Here's how the part is built. I have some questions about the finished solid (model axes, mm). Face numbers are marked on the shaded views. A direction names the side the tool comes from. Coordinates: 2 decimals unless noted, no trailing zeros. Order: outer loops, then holes, each group sorted by start corner. A loop starts at its lowest first (then second) coordinate and runs counter-clockwise, first axis right, second up. Notation, with made-up numbers: (23.25, 27.5) - (38.25, 27.5) arc R28 cw to (38.25, 48.5) - close; hole circle Ø10 at (85, -3). An arc over 180 degrees is marked (long way). Answer in a Markdown table with one row per item. Add a question column.
Item 1: Thinking about a two-plate mould opening in Y: for the marked faces 1, 2 and 3, which applies, +Y half, -Y half, draft (parallel to the pull), parting line (faces both ways), or undercut?
Item 2: On a 3-axis mill with a long thin cutter (end or side, diameter ignored), from which of +Z, -Z, +X, -X, +Y, -Y can I reach the whole of each face in a straight line? I mean the marked faces 4 and 5. Say none if no direction works.
Item 3: I want a section at D-D (y = 19.05). Please give me the cut outline in (x, z) (3 decimals), plus the area to 3 significant figures.
Item 4: If I drill on line 1 along Y through (x, z) = (26.5, -3) (3 decimals); line 2 along Z through (x, y) = (1, -0.5) (3 decimals); line 3 along X through (y, z) = (3.5, 2.5), over which ranges is the centre line in solid material (lowest first)? Write a range as from..to.
Item 5: I want a section at A-A (x = -7). Please give me the cut outline in (y, z) (3 decimals).
Item 6: I want a section at B-B (x = -25.4). Please give me the cut outline in (y, z) (1 decimal).
Item 7: I want a section at C-C (y = 4). Please give me the cut outline in (x, z) (3 decimals), plus the area to 3 significant figures.
Item 8: Will these pins go through, and if not, where does the flat tip stop? pin 1 Ø2 at (x, z) = (19.05, -2.38) entering from +Y; pin 2 Ø1.6 at (y, z) = (-29.5, -1.5) entering from -X (3 decimals); pin 3 Ø4.5 at (x, y) = (-25.4, 19.05) entering from -Z (3 decimals); pin 4 Ø3 at (x, z) = (19.05, -2.38) entering from -Y.
```python
from build123d import *

# Parameters (mm, degrees)
SKETCH1_W                 = 63.5
SKETCH1_H                 = 63.5
BOSS_EXTRUDE1_DEPTH       = 3.175
BOSS_EXTRUDE2_DEPTH       = 4.7625
F_2_CLEARANCE_HOLE1_D     = 2.4384
F_2_CLEARANCE_HOLE1_DEPTH = 3.175
FILLET1_R                 = 19.05
SKETCH5_W                 = 15.875
SKETCH5_H                 = 3.175
BOSS_EXTRUDE3_DEPTH       = 4.7625
F_2_CLEARANCE_HOLE2_D     = 2.4384
F_2_CLEARANCE_HOLE2_DEPTH = 3.175
BOSS_EXTRUDE4_START       = -3.175
SKETCH8_R                 = 3.175
BOSS_EXTRUDE4_DEPTH       = 3.175
F_6_CLEARANCE_HOLE1_D     = 3.7973
CUT_EXTRUDE1_REACH        = 9.938
SKETCH11_R                = 3.175


with BuildPart() as part:
    # Sketch1 → Boss-Extrude1 (new body)
    with BuildSketch(Plane.XY):
        Rectangle(SKETCH1_W, SKETCH1_H)
    extrude(amount=BOSS_EXTRUDE1_DEPTH)

    # Sketch2 → Boss-Extrude2 (add)
    with BuildSketch(Plane(origin=(0, 0, 0), x_dir=(-1, 0, 0), z_dir=(0, 0, -1))):
        Polygon((-25.4, -31.75), (-15.875, -31.75), (-15.875, -28.575), (-25.4, -28.575), (-31.75, -28.575), (-31.75, -31.75), align=None)
    extrude(amount=BOSS_EXTRUDE2_DEPTH)

    # #2 Clearance Hole1
    with Locations(Plane(origin=(0, -28.575, 0), x_dir=(1, 0, 0), z_dir=(0, 1, 0))):
        with Locations((28.575, 2.38125), (19.05, 2.38125)):
            Hole(F_2_CLEARANCE_HOLE1_D / 2, depth=F_2_CLEARANCE_HOLE1_DEPTH)

    # Fillet1
    fillet1_edges = [part.edges().sort_by_distance(p)[0] for p in [
        (-31.75, -31.75, 1.5875),
        (-31.75, 31.75, 1.5875),
    ]]
    fillet(fillet1_edges, radius=FILLET1_R)

    # Sketch5 → Boss-Extrude3 (add)
    with BuildSketch(Plane(origin=(0, 0, 0), x_dir=(-1, 0, 0), z_dir=(0, 0, -1))):
        with Locations((-23.8125, 30.1625)):
            Rectangle(SKETCH5_W, SKETCH5_H)
    extrude(amount=BOSS_EXTRUDE3_DEPTH)

    # #2 Clearance Hole2
    with Locations(Plane(origin=(0, 28.575, 0), x_dir=(-1, 0, 0), z_dir=(0, -1, 0))):
        with Locations((-19.05, 2.38125), (-28.575, 2.38125)):
            Hole(F_2_CLEARANCE_HOLE2_D / 2, depth=F_2_CLEARANCE_HOLE2_DEPTH)

    # Sketch8 → Boss-Extrude4 (add)
    with BuildSketch(Plane.XY.offset(3.175).offset(BOSS_EXTRUDE4_START)):
        with Locations((-25.4, 19.05)):
            Circle(SKETCH8_R)
        with Locations((-25.4, -14.2875)):
            Circle(SKETCH8_R)
        with Locations((22.225, 19.05)):
            Circle(SKETCH8_R)
        with Locations((8.73125, -24.209375)):
            Circle(SKETCH8_R)
        with Locations((-11.90625, -24.209375)):
            Circle(SKETCH8_R)
    extrude(amount=-BOSS_EXTRUDE4_DEPTH)

    # #6 Clearance Hole1 (through all)
    with Locations(Plane(origin=(0, 0, -3.175), x_dir=(-1, 0, 0), z_dir=(0, 0, -1))):
        with Locations((-22.225, 19.05), (25.4, 19.05), (25.4, -14.2875), (11.90625, -24.209375), (-8.73125, -24.209375)):
            Hole(F_6_CLEARANCE_HOLE1_D / 2)

    # Sketch11 → Cut-Extrude1 (cut, up to next)
    with BuildSketch(Plane.XY.offset(3.175), mode=Mode.PRIVATE) as cut_extrude1_sk1:
        with Locations((-1.5875, -23.415625)):
            Circle(SKETCH11_R)
    cut_extrude1_tool1 = extrude(cut_extrude1_sk1.sketch, amount=-CUT_EXTRUDE1_REACH, mode=Mode.PRIVATE) & part.part
    add(cut_extrude1_tool1.solids().sort_by_distance((-1.5875, -23.415625, 3.175))[0], mode=Mode.SUBTRACT)
    # Sketch11 → Cut-Extrude1 (cut, up to next)
    with BuildSketch(Plane.XY.offset(3.175), mode=Mode.PRIVATE) as cut_extrude1_sk2:
        with BuildLine():
            Line((-4.7625, 23.01875), (1.5875, 23.01875))
            ThreePointArc((1.5875, 23.01875), (12.7, 11.90625), (1.5875, 0.79375))
            Line((1.5875, 0.79375), (-4.7625, 0.79375))
            ThreePointArc((-4.7625, 0.79375), (-15.875, 11.90625), (-4.7625, 23.01875))
        make_face()
    cut_extrude1_tool2 = extrude(cut_extrude1_sk2.sketch, amount=-CUT_EXTRUDE1_REACH, mode=Mode.PRIVATE) & part.part
    add(cut_extrude1_tool2.solids().sort_by_distance((-1.5875, 11.90625, 3.175))[0], mode=Mode.SUBTRACT)


solid = part.part
```
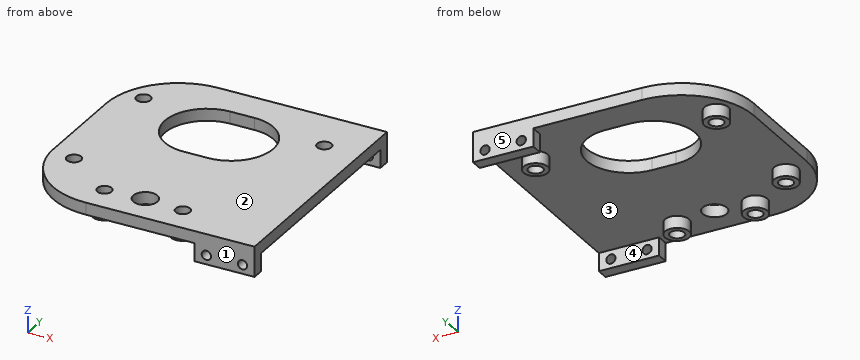
Values follow:
| question | item | result |
|---|---|---|
| 1 | face 1 | -Y half |
| 1 | face 2 | draft |
| 1 | face 3 | undercut |
| 2 | face 4 | -Z, +X, -X |
| 2 | face 5 | +Z, -Z, +X, -X, +Y |
| 3 | outline | (-30.661, 0) - (-28.575, 0) - (-28.575, -3.175) - (-27.299, -3.175) - (-27.299, 3.175) - (-30.661, 3.175) - close; (-23.501, -3.175) - (-22.225, -3.175) - (-22.225, 0) - (-13.275, 0) - (-13.275, 3.175) - (-23.501, 3.175) - close; (10.1, 0) - (19.05, 0) - (19.05, -3.175) - (20.326, -3.175) - (20.326, 3.175) - (10.1, 3.175) - close; (24.124, -3.175) - (25.4, -3.175) - (25.4, 0) - (31.75, 0) - (31.75, 3.175) - (24.124, 3.175) - close |
| 3 | area | 116 mm^2 |
| 4 | line 1 | y = -31.75..-28.575, 28.575..31.75 |
| 4 | line 2 | z = 0..3.175 |
| 4 | line 3 | x = -31.75..-12.03, 8.86..31.75 |
| 5 | outline | (-31.75, 0) - (1.021, 0) - (1.021, 3.175) - (-31.75, 3.175) - close; (22.791, 0) - (31.75, 0) - (31.75, 3.175) - (22.791, 3.175) - close |
| 6 | outline | (-26.9, 0) - (-17.5, 0) - (-17.5, -3.2) - (-16.2, -3.2) - (-16.2, 3.2) - (-26.9, 3.2) - close; (-12.4, -3.2) - (-11.1, -3.2) - (-11.1, 0) - (15.9, 0) - (15.9, -3.2) - (17.2, -3.2) - (17.2, 3.2) - (-12.4, 3.2) - close; (20.9, -3.2) - (22.2, -3.2) - (22.2, 0) - (26.9, 0) - (26.9, 3.2) - (20.9, 3.2) - close |
| 7 | outline | (-31.75, 0) - (-12.571, 0) - (-12.571, 3.175) - (-31.75, 3.175) - close; (9.396, 0) - (31.75, 0) - (31.75, 3.175) - (9.396, 3.175) - close |
| 7 | area | 132 mm^2 |
| 8 | pin 1 | stops at y = 21.36 |
| 8 | pin 2 | stops at x = 15.875 |
| 8 | pin 3 | stops at z = -3.175 |
| 8 | pin 4 | stops at y = -31.75 |
